Study the drawing (mm; zero at the part's minimum x, y, z) and answer. A direction names the side the tool comes from. Coordinates: 2 decimals unless noted, no trailing zeros. Loops run counter-clockwise (first coordinate to the right, second up) from the corner with the lowest first, then second, coordinate; pieces in that order, holes last.
Q1. Which of the six approach directions +Z, -Z, +X, -X, +Y, -Y give full straight-line access (tool end or side, diameter ignored) to the marked faces 1 and 2?
Q2. Section A-A (y = 60) is taken. Give the vertices of the cut face in (x, z), then the cut area to 4 significant figures.
Q3. Section C-C (z = 30) is taken. Give the vertices of the cut face in (x, y), then the cut area to 3 significant figures.
Q4. Flat-ended cylindrical pins translate along their axes: P1, Ø10, axis at x = 28, y = 57.5, coming from the +Z side; P2, Ø10, axis at x = 20, y = 58, coming from the +Z side; P3, Ø2, axis at x = 5, y = 13, coming from the +Z side; P4, Ø13, axis at x = 30, y = 20, coming from the -Z side. Find the tip coordinate at first contact, or state that the pin passes through.
Q5. Section B-B (x = 30) is taken. Give the vertices of the cut face in (y, z).
Q6. Straight lines are drawn through the part: line 1 (Y direction, x = 30, z = 1.7); line 2 (Z direction, x = 1.3, y = 20). For each, find the intervals that lie inside material, in ascending order.
Q7. Section D-D (y = 43.5) is taken. Give the vertices of the cut face in (x, z), then the cut area to 4 significant figures.
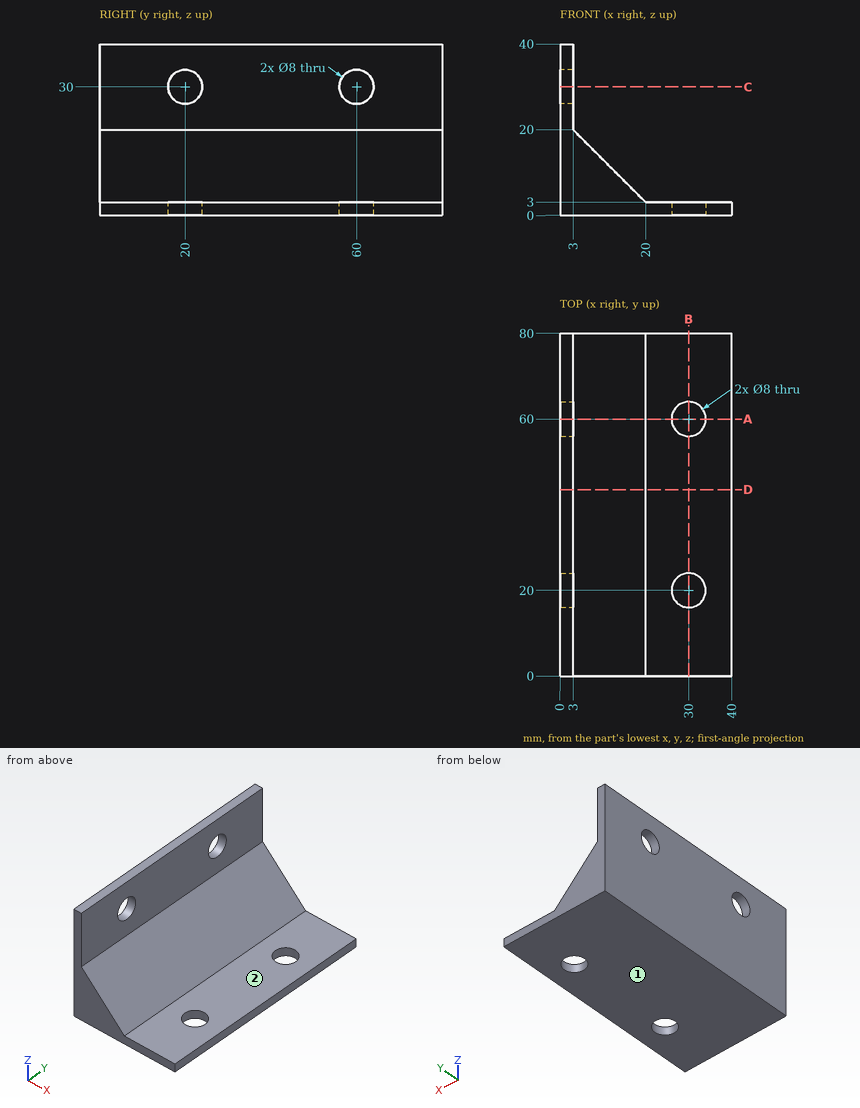
Numbers:
1. face 1: -Z, +X, -X, +Y, -Y
1. face 2: +Z, +X, +Y, -Y
2. outline: (0, 0) - (26, 0) - (26, 3) - (20, 3) - (3, 20) - (3, 26) - (0, 26) - close; (0, 34) - (3, 34) - (3, 40) - (0, 40) - close; (34, 0) - (40, 0) - (40, 3) - (34, 3) - close
2. area: 327.5 mm2
3. outline: (0, 0) - (3, 0) - (3, 16) - (0, 16) - close; (0, 24) - (3, 24) - (3, 56) - (0, 56) - close; (0, 64) - (3, 64) - (3, 80) - (0, 80) - close
3. area: 192 mm2
4. P1: stops at z = 3
4. P2: stops at z = 8
4. P3: stops at z = 19
4. P4: stops at z = 0
5. outline: (0, 0) - (16, 0) - (16, 3) - (0, 3) - close; (24, 0) - (56, 0) - (56, 3) - (24, 3) - close; (64, 0) - (80, 0) - (80, 3) - (64, 3) - close
6. line 1: y = 0 to 16, 24 to 56, 64 to 80
6. line 2: z = 0 to 26, 34 to 40
7. outline: (0, 0) - (40, 0) - (40, 3) - (20, 3) - (3, 20) - (3, 40) - (0, 40) - close
7. area: 375.5 mm2
